Job drawing, mm, ordinate dimensions from the low corner. One solid piece. A direction names the side the tool comes from. Give positions to 0.01 mm unless a question says otherwise; leave off trailing zeros. Loops run counter-clockwise (first coordinate to the right, second up) from the corner with the lowest first, then second, coordinate; pieces in that order, holes last. Notation, with made-up numbers: M -2.75,19 L 22.25,19 A19 ccw 22.25,55 Z; hole C 66,49.5 d3. An arc over 180 degrees is marked long. Answer in a Markdown table with one row per item.
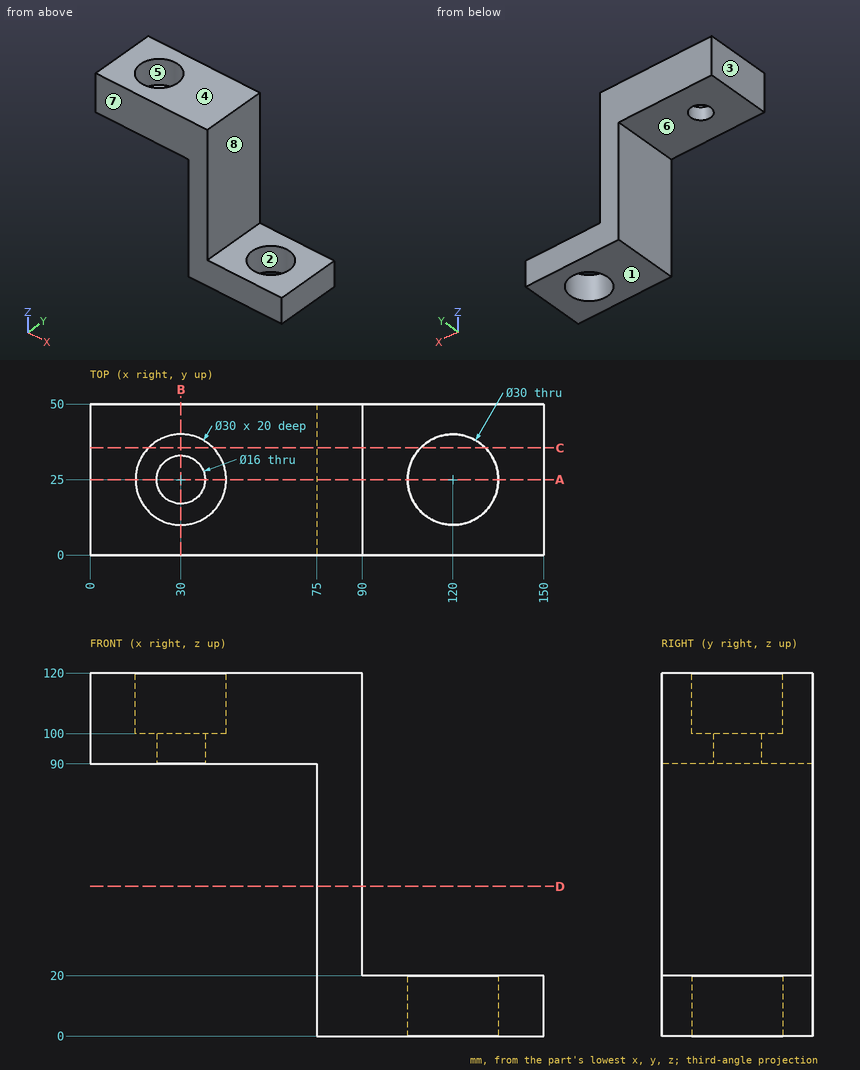
(1) Saw through at D-D (z = 49.5). Write the cut outline in (x, y), plus the area to 3 significant figures.
Recorded:
| item | result |
|---|---|
| outline | M 75,0 L 90,0 L 90,50 L 75,50 Z |
| area | 750 mm^2 |
(2) Which spindle directions (+Z, -Z, +X, -X, +Y, -Y) get a long thin tool onto all of the face, cutting with end or side? Do the marked faces 4, 5, 6, 7 and 8. Say none if no direction does.
Recorded:
| item | result |
|---|---|
| face 4 | +Z, +X, -X, +Y, -Y |
| face 5 | +Z |
| face 6 | -Z, -X, +Y, -Y |
| face 7 | +Z, -Z, +X, -X, -Y |
| face 8 | +Z, +X, +Y, -Y |
(3) Pull direction X, two halves, no side cores. Call the marked faces 1, 2 and 3: +X half, -X half, draft (parallel to the pull), parting line (faces both ways), or undercut.
Recorded:
| item | result |
|---|---|
| face 1 | draft |
| face 2 | undercut |
| face 3 | -X half |
(4) Saw through at A-A (y = 25). Write the cut outline in (x, z), plus the area to 3 significant figures.
Recorded:
| item | result |
|---|---|
| outline | M 0,90 L 22,90 L 22,100 L 15,100 L 15,120 L 0,120 Z; M 38,90 L 75,90 L 75,0 L 105,0 L 105,20 L 90,20 L 90,120 L 45,120 L 45,100 L 38,100 Z; M 135,0 L 150,0 L 150,20 L 135,20 Z |
| area | 3,890 mm^2 |
(5) Saw through at B-B (x = 30). Write the cut outline in (y, z).
Recorded:
| item | result |
|---|---|
| outline | M 0,90 L 17,90 L 17,100 L 10,100 L 10,120 L 0,120 Z; M 33,90 L 50,90 L 50,120 L 40,120 L 40,100 L 33,100 Z |
(6) Drill centre lines: line 1 along Y through (x, z) = (30, 106); line 2 along X through (y, z) = (25, 9.75); line 3 along Y through (x, z) = (30, 93). Where is each one in solid material? Low to high.
Recorded:
| item | result |
|---|---|
| line 1 | y = 0 to 10, 40 to 50 |
| line 2 | x = 75 to 105, 135 to 150 |
| line 3 | y = 0 to 17, 33 to 50 |
(7) Saw through at C-C (y = 35.5). Write the cut outline in (x, z), plus the area to 3 significant figures.
Recorded:
| item | result |
|---|---|
| outline | M 0,90 L 75,90 L 75,0 L 109.29,0 L 109.29,20 L 90,20 L 90,120 L 40.71,120 L 40.71,100 L 19.29,100 L 19.29,120 L 0,120 Z; M 130.71,0 L 150,0 L 150,20 L 130.71,20 Z |
| area | 4,390 mm^2 |
(8) Pin check, flat tips, straight feed: pin 1 Ø1.5 at (x, y) = (22, 44.5) entering from -Z; pin 2 Ø4 at (y, z) = (35.5, 87.5) entering from +X; pin 3 Ø25 at (y, z) = (15, 62.5) entering from -X. Stop position of each tip, or through.
Recorded:
| item | result |
|---|---|
| pin 1 | stops at z = 90 |
| pin 2 | stops at x = 90 |
| pin 3 | stops at x = 75 |
